Build history of the part. All positions in model axes, mm. A direction names the side the tool comes from. Round coordinates to 2 decimals unless told otherwise and drop trailing zeros. Write each loop counter-clockwise with the first axis right and the second up, starting at its lowest first coordinate (ties: lowest second). Pieces come first, ordered by that corner, then holes.
1) Saw through at B-B (z = 89.5). Write the cut outline in (x, y).
2) Saw through at A-A (z = 15). Write the cut outline in (x, y), plus the area to 3 significant figures.
3) Which spindle directions (+Z, -Z, +X, -X, +Y, -Y) get a long thin tool onto all of the face, cutting with end or side? Do faces 4 (the flat face through (48.551, -14.989, 44.427)), 5 (the flat face through (110, 19, 15)), 6 (the flat face through (72, 19.5, 57)), 7 (the flat face through (74.35, 9.37, 78.38)). Say none if no direction does.
4) Flat gauge pins, fed straight in: pin 1 (4 mm diameter, centred on x = 88.8, z = 15, fed in from +Y); pin 2 (8.5 mm diameter, centred on x = 57.5, z = 36, fed in from -Y); pin 3 (10 mm diameter, centred on x = 120.5, y = 8, fed in from +Z); pin 4 (12 mm diameter, centred on x = 61.5, y = 13, fed in from +Z). Where does each tip first touch, or does it go through?
5) Wall check: probe 1 along Z at (x, y) = (113, 18); probe 2 along Z at (x, y) = (95, 8); probe 3 along X at (y, z) = (21.65, 15). Give the ranges that are in metal, low to high.
6) Pull direction X, two halves, no side cores. Call faces 1 (the flat face through (68.917, -12.686, 39.547)), 2 (the flat face through (71, 0, 41)), 3 (the flat face through (49.56, -0.72, 40.39)): +X half, -X half, draft (parallel to the pull), parting line (faces both ways), or undercut.
7) Saw through at C-C (z = 73.5). Write the cut outline in (x, y).
from build123d import *

# Parameters (mm, degrees)
BOSS_EXTRUDE1_DEPTH      = 23
SKETCH2_W                = 100.39999999999999
SKETCH2_H                = 20.400000000000002
CUT_EXTRUDE2_DEPTH       = 19
CUT_EXTRUDE3_DEPTH       = 19
CUT_EXTRUDE11_DEPTH      = 200.75985582694003
CUT_EXTRUDE11_DEPTH_BACK = 200.75985582694003
CUT_EXTRUDE10_DEPTH      = 20
SKETCH38_R               = 2.299999999999993
SKETCH38_R_2             = 2.300000000000006
SKETCH38_R_3             = 2.2999999999999985
SKETCH38_R_4             = 2.299999999999992
CUT_EXTRUDE24_DEPTH      = 10
BOSS_EXTRUDE2_DEPTH      = 6
SKETCH40_R               = 1.6500000000000017
CUT_EXTRUDE25_DEPTH      = 200.1582285520733
SKETCH41_R               = 3.0000000000000084
CUT_EXTRUDE26_DEPTH      = 3.5
SKETCH45_R               = 2.3
CUT_EXTRUDE29_DEPTH      = 130.1236252028075
SKETCH47_R               = 7.499999999999999
CUT_EXTRUDE31_DEPTH      = 10
CUT_EXTRUDE32_DEPTH      = 200.75985582694003
BOSS_EXTRUDE3_DEPTH      = 21
CUT_EXTRUDE33_DEPTH      = 200.75985582694003
CHAMFER6_SIZE            = 0.8
CHAMFER6_SIZE2           = 9.144041842209413
SKETCH51_R               = 4.5
CUT_EXTRUDE34_DEPTH      = 29.803050969
SKETCH52_R               = 2.3
CUT_EXTRUDE35_DEPTH      = 10
SKETCH53_W               = 20.000000000000007
SKETCH53_H               = 20
CUT_EXTRUDE36_DEPTH      = 10
SKETCH54_R               = 0.8500000000000069
CUT_EXTRUDE37_DEPTH      = 10
CHAMFER7_SIZE            = 1
CHAMFER7_SIZE_2          = 1.710027066
CHAMFER5_SIZE            = 14.54
CHAMFER4_SIZE            = 14.54


with BuildPart() as part:
    # Sketch1 → Boss-Extrude1 (new body)
    with BuildSketch(Plane(origin=(0, 0, 0), x_dir=(1, 0, 0), z_dir=(0, 1, 0))):
        Polygon((0, 0), (149.99999999999937, 0), (74.99999999999966, 129.903810567666), align=None)
    extrude(amount=BOSS_EXTRUDE1_DEPTH)

    # Sketch2 → Cut-Extrude2 (cut)
    with BuildSketch(Plane(origin=(0, 0, 0), x_dir=(1, 0, 0), z_dir=(0, 1, 0))):
        Polygon((108.9238401753675, 138.2616253392494), (58.72384017536752, 51.31267479929176), (41.05692193816496, 61.51267479929177), (91.25692193816495, 148.4616253392494), align=None)
        with Locations((124, 15.000000000000002)):
            Rectangle(SKETCH2_W, SKETCH2_H)
    extrude(amount=CUT_EXTRUDE2_DEPTH, mode=Mode.SUBTRACT)

    # Sketch4 → Cut-Extrude3 (cut)
    with BuildSketch(Plane(origin=(0, 0, 0), x_dir=(1, 0, 0), z_dir=(0, 1, 0))):
        Polygon((58.51558394542647, 45.56193363414623), (40.84866570822394, 35.36193363414623), (51.048665708223936, 17.69501539694368), (68.71558394542647, 27.895015396943673), align=None)
    extrude(amount=CUT_EXTRUDE3_DEPTH, mode=Mode.SUBTRACT)

    # Sketch22 → Cut-Extrude11 (cut, two sides: drawn at the far end of the back side and taken through both)
    with BuildSketch(Plane.XZ.offset(-CUT_EXTRUDE11_DEPTH_BACK)):
        Polygon((79.88924971530794, -26.147760514529192), (62.58924971530795, -56.11223948547077), (80.77578319478118, -66.61223948547077), (98.07578319478117, -36.64776051452918), align=None)
    extrude(amount=CUT_EXTRUDE11_DEPTH + CUT_EXTRUDE11_DEPTH_BACK, mode=Mode.SUBTRACT)

    # Sketch21 → Cut-Extrude10 (cut)
    with BuildSketch(Plane.XZ):
        Polygon((132.67949192431067, -29.999999999999993), (105.37797113249052, -29.999999999999993), (78.6697476797782, -76.26000000000042), (92.32050807568827, -99.90381056766569), align=None)
    extrude(amount=-CUT_EXTRUDE10_DEPTH, mode=Mode.SUBTRACT)

    # Sketch38 → Cut-Extrude24 (cut)
    with BuildSketch(Plane.XZ.offset(-19)):
        with Locations(Location((88.79999999999998, -15, 0), (0, 0, 270))):
            Circle(SKETCH38_R)
        with Locations(Location((123.8, -15, 0), (0, 0, 270))):
            Circle(SKETCH38_R_2)
        with Locations(Location((57.390381056766245, -69.40305585605834, 0), (0, 0, 270))):
            Circle(SKETCH38_R_3)
        with Locations(Location((74.89038105676623, -99.7139449885137, 0), (0, 0, 270))):
            Circle(SKETCH38_R_4)
    extrude(amount=-CUT_EXTRUDE24_DEPTH, mode=Mode.SUBTRACT)

    # Sketch39 → Boss-Extrude2 (add)
    with BuildSketch(Plane(origin=(0, 23, 0), x_dir=(1, 0, 0), z_dir=(0, 1, 0))):
        Polygon((62.58924971530795, 56.11223948547077), (80.77578319478118, 66.61223948547077), (84.77578319478118, 59.68403625519526), (66.58924971530797, 49.18403625519524), align=None)
        Polygon((98.07578319478117, 36.64776051452918), (79.88924971530794, 26.147760514529192), (75.88924971530795, 33.0759637448047), (94.07578319478117, 43.575963744804696), align=None)
    extrude(amount=-BOSS_EXTRUDE2_DEPTH)

    # Sketch40 → Cut-Extrude25 (cut, through all)
    with BuildSketch(Plane.XZ.offset(-17)):
        with Locations(Location((87.08251645504455, -34.68865704891005, 0), (0, 0, 270))):
            Circle(SKETCH40_R)
        with Locations(Location((73.58251645504457, -58.071342951089896, 0), (0, 0, 270))):
            Circle(SKETCH40_R)
    extrude(amount=-CUT_EXTRUDE25_DEPTH, mode=Mode.SUBTRACT)

    # Sketch41 → Cut-Extrude26 (cut)
    with BuildSketch(Plane(origin=(0, 23, 0), x_dir=(1, 0, 0), z_dir=(0, 1, 0))):
        with Locations(Location((73.58251645504457, 58.071342951089896, 0), (0, 0, 270))):
            Circle(SKETCH41_R)
        with Locations(Location((87.08251645504455, 34.68865704891005, 0), (0, 0, 270))):
            Circle(SKETCH41_R)
    extrude(amount=-CUT_EXTRUDE26_DEPTH, mode=Mode.SUBTRACT)

    # Sketch45 → Cut-Extrude29 (cut, through all)
    with BuildSketch(Plane(origin=(63.615583945425506, 0, -36.72847451554663), x_dir=(0.5, 0, 0.8660254037844386), z_dir=(-0.8660254037844387, 0, 0.5000000000000001))):
        with Locations((1.94809e-12, 9.5)):
            Circle(SKETCH45_R)
    extrude(amount=-CUT_EXTRUDE29_DEPTH, mode=Mode.SUBTRACT)

    # Sketch47 → Cut-Extrude31 (cut)
    with BuildSketch(Plane.XZ.offset(-19)):
        with Locations(Location((54.78212482682521, -31.62847451554496, 0), (0, 0, 270))):
            Circle(SKETCH47_R)
    extrude(amount=-CUT_EXTRUDE31_DEPTH, mode=Mode.SUBTRACT)

    # Sketch48 → Cut-Extrude32 (cut, through all)
    with BuildSketch(Plane.XZ):
        Polygon((55.491384919067684, 2e-17), (27.74569245953363, -48.05694903109369), (0, 0), align=None)
    extrude(amount=-CUT_EXTRUDE32_DEPTH, mode=Mode.SUBTRACT)

    # Sketch49 → Boss-Extrude3 (add)
    with BuildSketch(Plane.XZ):
        Polygon((48.718538689301745, -11.730913781805928), (75.91173636813312, -27.430913781805906), (61.7117363681331, -52.026035249283986), (34.51853868930174, -36.326035249284), align=None)
    extrude(amount=BOSS_EXTRUDE3_DEPTH)

    # Sketch50 → Cut-Extrude33 (cut, through all)
    with BuildSketch(Plane(origin=(0, 0, 0), x_dir=(1, 0, 0), z_dir=(0, 1, 0))):
        Polygon((40.84866570822394, 35.36193363414623), (58.51558394542647, 45.56193363414623), (68.71558394542649, 27.895015396943673), (51.048665708223936, 17.69501539694368), align=None)
    extrude(amount=-CUT_EXTRUDE33_DEPTH, mode=Mode.SUBTRACT)

    # Chamfer6
    chamfer6_edges = [part.edges().sort_by_distance(p)[0] for p in [
        (48.115137528717426, 0, -44.17603524928399),
        (62.31513752871743, 0, -19.58091378180592),
    ]]
    chamfer6_side = [part.faces().sort_by_distance(p)[0] for p in [
        (48.99845735329998, 0, -54.86781762841321),
    ]]
    chamfer(chamfer6_edges, length=CHAMFER6_SIZE, length2=CHAMFER6_SIZE2, reference=chamfer6_side[0])

    # Sketch51 → Cut-Extrude34 (cut)
    with BuildSketch(Plane(origin=(92.02385940613446, 0, -53.129999999999995), x_dir=(-0.4999999999999997, 0, -0.8660254037844388), z_dir=(0.8660254037844388, 0, -0.4999999999999997))):
        with Locations(Location((-1.92901e-12, 9.5, 0), (0, 0, 180))):
            Circle(SKETCH51_R)
    extrude(amount=-CUT_EXTRUDE34_DEPTH, mode=Mode.SUBTRACT)

    # Sketch52 → Cut-Extrude35 (cut)
    with BuildSketch(Plane(origin=(68.8117363681321, 0, -39.72847451554662), x_dir=(-0.49999999999999983, 0, -0.8660254037844387), z_dir=(0.8660254037844387, 0, -0.49999999999999983))):
        with Locations((-1.388e-14, -10)):
            Circle(SKETCH52_R)
    extrude(amount=-CUT_EXTRUDE35_DEPTH, mode=Mode.SUBTRACT)

    # Sketch53 → Cut-Extrude36 (cut)
    with BuildSketch(Plane(origin=(7.10000000000096, 0, 12.297560733740706), x_dir=(0.8660254037844387, 0, -0.49999999999999983), z_dir=(0.49999999999999983, 0, 0.8660254037844387))):
        with Locations((69.45694903109329, -11)):
            Rectangle(SKETCH53_W, SKETCH53_H)
    extrude(amount=CUT_EXTRUDE36_DEPTH, mode=Mode.SUBTRACT)

    # Sketch54 → Cut-Extrude37 (cut)
    with BuildSketch(Plane(origin=(7.10000000000096, 0, 12.297560733740706), x_dir=(0.8660254037844387, 0, -0.49999999999999983), z_dir=(0.49999999999999983, 0, 0.8660254037844387))):
        with Locations((64.5819490310929, -13.3999999999983)):
            Circle(SKETCH54_R)
        with Locations((74.58194903109292, -13.399999999998368)):
            Circle(SKETCH54_R)
    extrude(amount=-CUT_EXTRUDE37_DEPTH, mode=Mode.SUBTRACT)

    # Chamfer7
    # the kernel refuses this chamfer: 1.710027066, 1 mm, written as the material it takes off along each edge
    with BuildSketch(Plane(origin=(80.10050658552632, -1.0000000000000009, -29.026564170563404), x_dir=(0.07067759261755262, 0.9899589444048419, 0.12241718137025635), z_dir=(-0.866025403784439, 0, 0.49999999999999933))) as chamfer7_piece_1_section:
        Polygon((CHAMFER7_SIZE * 0.998511767905, CHAMFER7_SIZE * 0.0545366789897), (-CHAMFER7_SIZE_2 * 0.141355185248, CHAMFER7_SIZE_2 * 0.989958944496), (0, 0), align=None)
    chamfer7_piece_1 = extrude(amount=24.42540661325694, mode=Mode.PRIVATE)
    chamfer7_piece_1 = split(chamfer7_piece_1, bisect_by=Plane(origin=(69.16773960486616, -0.5972584462527297, -23.537265435119764), z_dir=(0.4999999999999995, 0, 0.866025403784439)), keep=Keep.TOP, mode=Mode.PRIVATE)
    add(chamfer7_piece_1, mode=Mode.SUBTRACT)

    # Chamfer5
    chamfer5_edges = [part.edges().sort_by_distance(p)[0] for p in [
        (55.491384919067684, 11.5, 2e-17),
    ]]
    chamfer(chamfer5_edges, length=CHAMFER5_SIZE)

    # Chamfer4
    chamfer4_edges = [part.edges().sort_by_distance(p)[0] for p in [
        (27.74569245953363, 11.5, -48.05694903109369),
    ]]
    chamfer(chamfer4_edges, length=CHAMFER4_SIZE)


with BuildPart() as body_2:
    # Mirror1: mirrored copy
    add(part.part.mirror(Plane.XY))


solid = body_2.part
Evaluation:
1. outline: (51.67, 0) - (57.22, 0) - (57.22, 19) - (80.77, 19) - (80.77, 0) - (86.31, 0) - (86.31, 20) - (98.33, 20) - (98.33, 23) - (51.67, 23) - close
2. outline: (46.83, -21) - (54.38, -21) - (54.38, -9.14) - (55.98, 0) - (73.8, 0) - (73.8, 19) - (86.5, 19) - (86.5, 23) - (46.83, 23) - close; (91.1, 19) - (121.5, 19) - (121.5, 23) - (91.1, 23) - close; (126.1, 19) - (141.34, 19) - (141.34, 23) - (126.1, 23) - close
2. area: 1,020 mm2
3. face 4: +Z, -X, -Y
3. face 5: +X, -Y
3. face 6: +Y
3. face 7: -Y
4. pin 1: passes through
4. pin 2: stops at y = 19
4. pin 3: stops at z = 30
4. pin 4: stops at z = 116.91
5. probe 1: z = 0 to 4.8, 25.2 to 30
5. probe 2: z = 0 to 4.8, 25.2 to 34.87, 41.98 to 47.98
5. probe 3: x = 46.83 to 86.5, 91.1 to 121.5, 126.1 to 141.34
6. face 1: +X half
6. face 2: draft
6. face 3: undercut
7. outline: (42.44, 0) - (47.98, 0) - (47.98, 19) - (71.53, 19) - (71.53, 0) - (80.26, 0) - (80.26, 20) - (107.56, 20) - (107.56, 23) - (42.44, 23) - close
